from build123d import *

# Parameters (mm, degrees)
SKETCH115_W             = 9
SKETCH115_H             = 28
PAD054_DEPTH            = 2.4
SKETCH116_W             = 5
SKETCH116_H             = 2.2
PAD055_DEPTH            = 2.5
SKETCH118_W             = 9
SKETCH118_H             = 2.2
PAD057_DEPTH            = 1.5
SKETCH119_R             = 4
PAD058_DEPTH            = 7
BODY014_PLACEMENT_ANGLE = 90


with BuildPart() as part:
    # Sketch115 → Pad054 (new body)
    with BuildSketch(Plane.XY):
        Rectangle(SKETCH115_W, SKETCH115_H)
    extrude(amount=PAD054_DEPTH)

    # Sketch116 → Pad055 (join)
    with BuildSketch(Plane.XY):
        with Locations((0, -7.3)):
            Rectangle(SKETCH116_W, SKETCH116_H)
    extrude(amount=-PAD055_DEPTH)

    # Sketch118 → Pad057 (join)
    with BuildSketch(Plane.XY.offset(-2.5)):
        with Locations((0, -7.3)):
            Rectangle(SKETCH118_W, SKETCH118_H)
    extrude(amount=-PAD057_DEPTH)

    # Sketch119 → Pad058 (join)
    with BuildSketch(Plane.XY):
        with Locations((0, 8.4)):
            Circle(SKETCH119_R)
    extrude(amount=-PAD058_DEPTH)


with BuildPart() as part_1:
    # Body014 placement: moved
    add(part.part.moved(Location((8.4, -12, 20.1))).rotate(Axis((8.4, -12, 20.1), (0, 0, 1)), BODY014_PLACEMENT_ANGLE))


solid = part_1.part
Verification items for the finished model (mm, model axes). A direction names the side the tool comes from. Give positions to 0.01 mm unless a question says otherwise; leave off trailing zeros. Order: outer loops, then holes, each group sorted by start corner. A loop starts at its lowest first (then second) coordinate and runs counter-clockwise, first axis right, second up. Notation, with made-up numbers: M 65,85.25 L 112,85.25 A28 cw 112,107.25 Z; hole C -9.5,58.25 d1. An arc over 180 degrees is marked long. Answer as a JSON object with one key per item and string values. Group by question number.
1) Cross-section at D-D (y = -12). Enter the section's corners in (x, z).
2) Cross-section at A-A (z = 19). Enter the section's corners in (x, y), then the cut area to 3 significant figures.
3) Mould release check, pull along X, two halves, no side actions. Record for faces 4 (the face through (16.8, -12, 18)), 5 (the face through (16, -12, 16.1)), 6 (the face through (11, -12, 20.1)): released by +X, released by -X, zero draft, split by the parting line, or undercut.
4) Access from +Z, -Z, +X, -X, +Y, -Y to the whole of each face (thin tool, end or side, straight path). Record for faces 1 (the face through (16, -16, 17.6)), 2 (the face through (16, -9, 17.6)), 3 (the face through (2.4, -15.2, 16.6)).
5) Depth check by flat-ended pin: pin 1 Ø3 at (x, y) = (4.5, -11) entering from -Z; pin 2 Ø2 at (y, z) = (-13.5, 18.5) entering from +X; pin 3 Ø2.5 at (x, y) = (16, -12) entering from -Z; pin 4 Ø1.1 at (x, z) = (15.5, 19.5) entering from -Y. Enter the tip coordinate at first touch or a pass-through.
6) Scan lines: line 1 along Z through (x, y) = (6, -14.25); line 2 along Z through (x, y) = (16.5, -13.5); line 3 along X through (y, z) = (-13.25, 14.25). Record each from-to range of solid material in increasing order. Write a range as [from, to].
7) Cross-section at B-B (y = -9). Enter the section's corners in (x, z).
8) Cross-section at C-C (x = 0). Enter the section's corners in (y, z), then the cut area to 3 significant figures.
Result sheet:
{
 "1": {"outline": "M -5.6,20.1 L -4,20.1 L -4,13.1 L 4,13.1 L 4,20.1 L 14.6,20.1 L 14.6,16.1 L 16.8,16.1 L 16.8,20.1 L 22.4,20.1 L 22.4,22.5 L -5.6,22.5 Z"},
 "2": {"outline": "C 0,-12 d8; M 14.6,-14.5 L 16.8,-14.5 L 16.8,-9.5 L 14.6,-9.5 Z", "area": "61.3 mm2"},
 "3": {"face 4": "released by +X", "face 5": "zero draft", "face 6": "undercut"},
 "4": {"face 1": "+X, -Y", "face 2": "+X, +Y", "face 3": "-Z"},
 "5": {"pin 1": "stops at z = 13.1", "pin 2": "stops at x = 16.8", "pin 3": "stops at z = 16.1", "pin 4": "stops at y = -14.5"},
 "6": {"line 1": "z = [20.1, 22.5]", "line 2": "z = [16.1, 22.5]", "line 3": "x = [-3.8, 3.8]"},
 "7": {"outline": "M -5.6,20.1 L -2.65,20.1 L -2.65,13.1 L 2.65,13.1 L 2.65,20.1 L 22.4,20.1 L 22.4,22.5 L -5.6,22.5 Z; M 14.6,16.1 L 16.8,16.1 L 16.8,17.6 L 14.6,17.6 Z"},
 "8": {"outline": "M -16.5,20.1 L -16,20.1 L -16,13.1 L -8,13.1 L -8,20.1 L -7.5,20.1 L -7.5,22.5 L -16.5,22.5 Z", "area": "77.6 mm2"}
}
